Model file for the job. Use its own axes, mm. Give positions to 0.01 mm unless a question says otherwise; leave off trailing zeros. Loops run counter-clockwise (first coordinate to the right, second up) from the corner with the lowest first, then second, coordinate; pieces in that order, holes last. Notation, with made-up numbers: (79.25, -8) - (118.25, -8) arc R14 cw to (118.25, 5) - close; hole circle Ø6 at (-36.75, 34.5). An arc over 180 degrees is marked (long way). Answer as CSV lines item,"result". Start each with the question number.
Item 1: Drill centre lines: L1, parallel to Y at x = 8.5, z = -16.5; L2, parallel to X at y = 62.5, z = -0.5; L3, parallel to X at y = 108.5, z = 4. Where is each one in solid material? Low to high. Write a range as from..to.
Item 2: Saw through at B-B on x = 0. Give the cut face in (y, z), plus the area to 4 significant figures.
Item 3: Pin check, flat tips, straight feed: pin 1 (1 mm diameter, centred on y = 107.5, z = -12, fed in from -X); pin 2 (12 mm diameter, centred on x = 1.5, y = 29, fed in from -Z); pin 3 (1.5 mm diameter, centred on x = -2.5, y = 109, fed in from +Z). Stop position of each tip, or through.
Item 4: Saw through at A-A on y = 16.5. Give the cut face in (x, z).
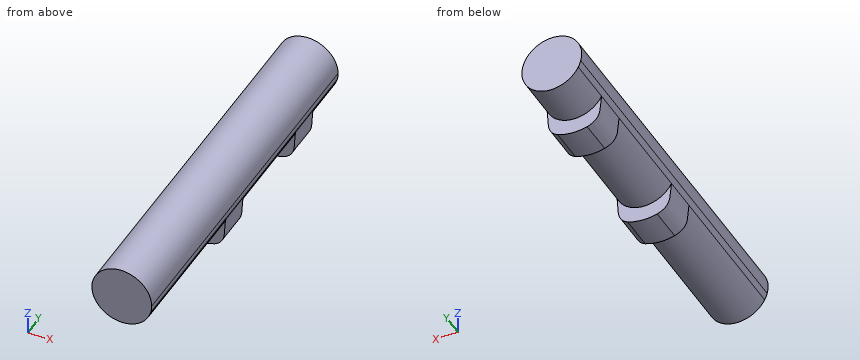
from build123d import *

# Parameters (mm, degrees)
SKETCH1_R           = 25.273
BOSS_EXTRUDE1_DEPTH = 203.2
CUT_EXTRUDE1_START  = -203.2
CUT_EXTRUDE1_DEPTH  = 203.2
SKETCH3_OUTSIDE_W   = 77.326
SKETCH3_OUTSIDE_H   = 85.949
SKETCH3_OUTSIDE_R   = 16.6497
CUT_EXTRUDE5_DEPTH  = 50.8
SKETCH4_OUTSIDE_W   = 77.326
SKETCH4_OUTSIDE_H   = 85.949
SKETCH4_OUTSIDE_R   = 16.6497
CUT_EXTRUDE6_DEPTH  = 57.15
SKETCH5_OUTSIDE_W   = 77.326
SKETCH5_OUTSIDE_H   = 85.949
SKETCH5_OUTSIDE_R   = 16.6497
CUT_EXTRUDE7_DEPTH  = 82.55


with BuildPart() as part:
    # Sketch1 → Boss-Extrude1 (new body)
    with BuildSketch(Plane(origin=(0, 0, 0), x_dir=(1, 0, 0), z_dir=(0, 1, 0))):
        with Locations(Location((0, 0, 0), (0, 0, 270))):
            Circle(SKETCH1_R)
    extrude(amount=BOSS_EXTRUDE1_DEPTH)

    # Sketch2 → Cut-Extrude1 (cut)
    with BuildSketch(Plane(origin=(0, 203.2, 0), x_dir=(1, 0, 0), z_dir=(0, 1, 0)).offset(CUT_EXTRUDE1_START)):
        with BuildLine():
            ThreePointArc((16.131428812, 4.121833886), (16.519624093, 2.077144651), (16.6497, 0))
            ThreePointArc((16.6497, 0), (-2.077144651, -16.519624093), (-16.131428812, 4.121833886))
            ThreePointArc((-16.131428812, 4.121833886), (-15.535644224, 5.988010406), (-14.724792916, 7.771292277))
            add(Edge.make_bspline(
                [(-14.724792916, 7.771292277), (-13.993112244, 11.833627294), (-14.951269099, 19.976611229), (-9.134694512, 23.553200783), (-6.765592548, 24.350591091)],
                knots=[0.117816193, 0.117816193, 0.117816193, 0.117816193, 0.459844437, 0.648405496, 0.648405496, 0.648405496, 0.648405496], degree=3))
            ThreePointArc((-6.765592548, 24.350591091), (-15.292771308, -20.121025688), (25.273, 0))
            ThreePointArc((25.273, 0), (21.007635157, 14.050046053), (9.651285593, 23.357594384))
            add(Edge.make_bspline(
                [(15.783143796, 5.301403776), (14.234187932, 11.657324188), (17.010518971, 19.800729125), (9.651285593, 23.357594384)],
                knots=[0.052591674, 0.052591674, 0.052591674, 0.052591674, 0.886528555, 0.886528555, 0.886528555, 0.886528555], degree=3))
            ThreePointArc((15.783143796, 5.301403776), (15.968181877, 4.714835907), (16.131428812, 4.121833886))
        make_face()
    extrude(amount=CUT_EXTRUDE1_DEPTH, mode=Mode.SUBTRACT)

    # Sketch3 outside → Cut-Extrude5 (cut)
    with BuildSketch(Plane(origin=(0, 177.8, 0), x_dir=(1, 0, 0), z_dir=(0, 1, 0))):
        with Locations((0, 4.3115)):
            Rectangle(SKETCH3_OUTSIDE_W, SKETCH3_OUTSIDE_H)
        with Locations(Location((0, 0, 0), (0, 0, 270))):
            Circle(SKETCH3_OUTSIDE_R, mode=Mode.SUBTRACT)
    extrude(amount=CUT_EXTRUDE5_DEPTH, mode=Mode.SUBTRACT)

    # Sketch4 outside → Cut-Extrude6 (cut)
    with BuildSketch(Plane(origin=(0, 101.6, 0), x_dir=(1, 0, 0), z_dir=(0, 1, 0))):
        with Locations((0, 4.3115)):
            Rectangle(SKETCH4_OUTSIDE_W, SKETCH4_OUTSIDE_H)
        with Locations(Location((0, 0, 0), (0, 0, 270))):
            Circle(SKETCH4_OUTSIDE_R, mode=Mode.SUBTRACT)
    extrude(amount=CUT_EXTRUDE6_DEPTH, mode=Mode.SUBTRACT)

    # Sketch5 outside → Cut-Extrude7 (cut)
    with BuildSketch(Plane(origin=(0, 0, 0), x_dir=(-1, 0, 0), z_dir=(0, -1, 0))):
        with Locations((0, 4.3115)):
            Rectangle(SKETCH5_OUTSIDE_W, SKETCH5_OUTSIDE_H)
        with Locations(Location((0, 0, 0), (0, 0, 270))):
            Circle(SKETCH5_OUTSIDE_R, mode=Mode.SUBTRACT)
    extrude(amount=-CUT_EXTRUDE7_DEPTH, mode=Mode.SUBTRACT)


solid = part.part
Responses:
1,L1,"82.55..101.6, 158.75..177.8"
1,L2,"-16.64..16.64"
1,L3,"-16.16..16.16"
2,outline,"(0, -16.65) - (82.55, -16.65) - (82.55, -25.27) - (101.6, -25.27) - (101.6, -16.65) - (158.75, -16.65) - (158.75, -25.27) - (177.8, -25.27) - (177.8, -16.65) - (203.2, -16.65) - (203.2, 16.65) - (0, 16.65) - close"
2,area,"7,095 mm2"
3,pin 1,"x = -12.04"
3,pin 2,"z = -16.65"
3,pin 3,"z = 16.56"
4,outline,"circle Ø33.3 at (0, 0)"
